Part model, mm, in its own coordinate system. A direction names the side the tool comes from. Round coordinates to 2 decimals unless told otherwise and drop trailing zeros. Write each loop counter-clockwise with the first axis right and the second up, starting at its lowest first coordinate (ties: lowest second). Pieces come first, ordered by that corner, then holes. Notation, with made-up numbers: M 5,-28.5 L 21,-28.5 A6 ccw 21,-20.5 Z; hole C 30,44 d2. An arc over 180 degrees is marked long. Use a Markdown table: item, result. Add a question column.
1) Which spindle directions (+Z, -Z, +X, -X, +Y, -Y) get a long thin tool onto all of the face, cutting with end or side? Do faces 1 (the face through (-12, 58, 5)), 2 (the face through (35, 30, -17)), 3 (the face through (-5, 30, -17)). Say none if no direction does.
2) Slice it at C-C on z = -20. Write the cut outline in (x, y), plus the area to 3 significant figures.
3) Slice it at B-B on z = -15. Write the cut outline in (x, y), plus the area to 3 significant figures.
4) Wall check: probe 1 along X at (y, z) = (58.5, -26.5); probe 2 along X at (y, z) = (30, 3.1); probe 3 along Z at (x, y) = (-10, 30). Give the ranges that are in metal, low to high.
5) Drop flat-ended pins along their axis: P1, Ø5.5, axis at y = 15, z = -15, coming from the -X side; P2, Ø1.5, axis at y = 23, z = -1.5, coming from the +X side; P3, Ø5, axis at x = 40.5, y = 2, coming from the +Z side; P4, Ø15, axis at x = 8.5, y = 19, coming from the -Z side. Give the stop position or say it passes through.
6) Two-plate mould, pull along Y, no slides. Class faces 4 (the face through (13, 0, 1)), 5 (the face through (15, 8, 0)), 6 (the face through (32.53, 17.57, -16.64)), 7 (the face through (15.3, 45.4, 5)): released by +Y, released by -Y, zero draft, split by the parting line, or undercut.
7) Slice it at A-A on x = 15. Write the cut outline in (y, z).
8) Slice it at D-D on z = 7. Write the cut outline in (x, y).
Autodesk Inventor part; units mm, degrees
ref_plane "YZ Plane" through (0, 0, 0) normal (1, 0, 0) x (0, 1, 0)
ref_plane "XZ Plane" through (0, 0, 0) normal (0, 1, 0) x (-1, 0, 0)
ref_plane "XY Plane" through (0, 0, 0) normal (0, 0, 1) x (1, 0, 0)
sketch "Sketch1" plane through (0, 0, 0) normal (0, 1, 0) x (-1, 0, 0)
  line L0 (0, 0) -> (-30, 0)
  line L1 (-30, 0) -> (-30, -30)
  line L2 (-30, -30) -> (0, -30)
  line L3 (0, -30) -> (0, 0)
  line L4 (-35, -35) -> (-35, 5)
  line L5 (-35, 5) -> (5, 5)
  line L6 (5, 5) -> (5, -35)
  line L7 (5, -35) -> (-35, -35)
  line L8 (0, -30) -> (5, -30)
  line L9 (-30, -30) -> (-35, -30)
  dimension "d0" = 30
  dimension "d1" = 30
  dimension "d2" = 5
extrude "Extrusion1" add sketch "Sketch1" along normal blind 60 contours L0 L1 L9 L4 L5 L6 L8 L3
sketch "Sketch2" plane through (-5, 0, 5) normal (0, 0, 1) x (1, 0, 0)
  line L0 (0, 0) -> (40, 0)
  line L1 (40, 0) -> (40, 60)
  line L2 (0, 60) -> (40, 60)
  line L3 (0, 0) -> (0, 60)
  line L4 (0, 60) -> (40, 60)
  line L5 (0, 0) -> (40, 0)
  line L6 (0, 60) -> (40, 0) construction
  circle A0 centre (20, 30) radius 23.6
  circle A1 centre (20, 30) radius 27.6
  dimension "d5" = 47.2
  dimension "d6" = 4
extrude "Extrusion2" add sketch "Sketch2" along normal blind 13 contours A1 L3 A0 | L3 A0 L1 A1 | L1 A0 A1 | A1 L1 A0 L3
sketch "Sketch3" plane through (35, 0, 5) normal (1, 0, 0) x (0, 0, -1)
  line L0 (5, 60) -> (35, 60)
  line L1 (35, 60) -> (0, 60)
  line L2 (5, 0) -> (35, 0)
  line L3 (0, 60) -> (4, 60)
  line L4 (4, 60) -> (4, 0)
  line L5 (4, 0) -> (0, 0)
  line L6 (0, 0) -> (0, 60)
  point P0 (4, 60)
  dimension "d10" = 4
extrude "Extrusion3" add sketch "Sketch3" along normal blind 9
sketch "Sketch4" plane through (-5, 0, -30) normal (-1, 0, 0) x (0, 0, 1)
  line L0 (0, 60) -> (35, 60)
  line L1 (30, 0) -> (0, 0)
  line L2 (35, 60) -> (30, 60)
  line L3 (30, 60) -> (30, 0)
  line L4 (30, 0) -> (35, 0)
  line L5 (35, 0) -> (35, 60)
extrude "Extrusion4" add sketch "Sketch4" along normal blind 9
sketch "Sketch5" plane through (15, 30, 5) normal (0, 0, 1) x (1, 0, 0)
  circle A0 centre (0, 0) radius 23.6
  circle A1 centre (0, 0) radius 15
  point P0 (-15, -30)
  dimension "d15" = 30
extrude "Extrusion5" cut sketch "Sketch5" against normal blind 9 contours A1
fillet "Fillet1" radius 10 1 edges at (-12.6, 30, 5)
sketch "Sketch7" plane through (35, 0, -30) normal (1, 0, 0) x (0, 0, -1)
  line L0 (-31, 60) -> (-31, 0)
  line L1 (-31, 0) -> (0, 0)
  line L2 (0, 0) -> (0, 60)
  line L3 (-31, 60) -> (0, 60)
  line L4 (-30, 0) -> (0, 0)
  line L5 (-15, 0) -> (-15, 15) construction
  line L6 (-15, 15) -> (-15, 45) construction
  line L7 (-15, 45) -> (-15, 60) construction
  line L8 (0, 60) -> (-31, 60)
  circle A0 centre (-15, 15) radius 3.05
  circle A1 centre (-15, 45) radius 3.05
  dimension "d19" = 30
  dimension "d20" = 6.1
extrude "Extrusion6" cut sketch "Sketch7" against normal blind 40 contours A0 | A1
fillet "Fillet2" radius 5 2 edges at (-5, 30, 0) (35, 30, 1)
properties part number "Bearing holder_3DPrint"
Entries:
| question | item | result |
|---|---|---|
| 1 | face 1 | +Z, -X, +Y |
| 1 | face 2 | -Z, +X, +Y, -Y |
| 1 | face 3 | -Z, -X, +Y, -Y |
| 2 | outline | M -5,0 L 0,0 L 0,60 L -5,60 Z; M 30,0 L 35,0 L 35,60 L 30,60 Z |
| 2 | area | 600 mm^2 |
| 3 | outline | M -5,0 L 0,0 L 0,11.95 L -5,11.95 Z; M -5,18.05 L 0,18.05 L 0,41.95 L -5,41.95 Z; M -5,48.05 L 0,48.05 L 0,60 L -5,60 Z; M 30,0 L 35,0 L 35,11.95 L 30,11.95 Z; M 30,18.05 L 35,18.05 L 35,41.95 L 30,41.95 Z; M 30,48.05 L 35,48.05 L 35,60 L 30,60 Z |
| 3 | area | 478 mm^2 |
| 4 | probe 1 | x = -5 to 0, 30 to 35 |
| 4 | probe 2 | x = -14 to 0, 30 to 44 |
| 4 | probe 3 | z = 0 to 18 |
| 5 | P1 | passes through |
| 5 | P2 | stops at x = 36.2 |
| 5 | P3 | stops at z = 5.25 |
| 5 | P4 | stops at z = 0 |
| 6 | face 4 | released by -Y |
| 6 | face 5 | zero draft |
| 6 | face 6 | undercut |
| 6 | face 7 | undercut |
| 7 | outline | M 0,0 L 15,0 L 15,5 L 6.4,5 L 6.4,18 L 2.4,18 L 2.4,15 A10 cw 0,8.5 Z; M 45,0 L 60,0 L 60,8.5 A10 cw 57.6,15 L 57.6,18 L 53.6,18 L 53.6,5 L 45,5 Z |
| 8 | outline | M -14,17.45 A31.6 ccw 5.07,0 L 24.93,0 A31.6 ccw 44,17.45 L 44,42.55 A31.6 ccw 24.93,60 L 5.07,60 A31.6 ccw -14,42.55 Z; hole C 15,30 d47.2 |
